from build123d import *

# Parameters (mm, degrees)
SKETCH_1_W          = 40
SKETCH_1_H          = 80
SKETCH_1_R          = 4.25
SKETCH_1_R_2        = 5.1
EXTRUDE_1_DEPTH     = 12
SKETCH_3_R          = 6.5
CUT_EXTRUDE_1_DEPTH = 7
SWEEP_1_PITCH       = 1.75
SWEEP_1_HEIGHT      = 12
SWEEP_1_RADIUS      = 5.1
SWEEP_1_START_ANGLE = 90
SKETCH_6_W          = 42.021889548
SKETCH_6_H          = 2.845778449
SKETCH_6_W_2        = 42.914668854
SKETCH_6_H_2        = 10.152042119
CUT_EXTRUDE_2_DEPTH = 91.331481783


with BuildPart() as part:
    # 草图1 → 凸台-拉伸1 (new body)
    with BuildSketch(Plane(origin=(0, 0, 0), x_dir=(1, 0, 0), z_dir=(0, 1, 0))):
        with Locations((20, 40)):
            Rectangle(SKETCH_1_W, SKETCH_1_H)
        with Locations(Location((20, 60, 0), (0, 0, 270))):
            Circle(SKETCH_1_R, mode=Mode.SUBTRACT)
        with Locations(Location((20, 20, 0), (0, 0, 270))):
            Circle(SKETCH_1_R, mode=Mode.SUBTRACT)
        with Locations(Location((20, 40, 0), (0, 0, 270))):
            Circle(SKETCH_1_R_2, mode=Mode.SUBTRACT)
    extrude(amount=EXTRUDE_1_DEPTH)

    # 草图3 → 切除-拉伸1 (cut)
    with BuildSketch(Plane(origin=(0, 12, 0), x_dir=(1, 0, 0), z_dir=(0, 1, 0))):
        with Locations(Location((20, 20, 0), (0, 0, 270))):
            Circle(SKETCH_3_R)
        with Locations(Location((20, 60, 0), (0, 0, 270))):
            Circle(SKETCH_3_R)
    extrude(amount=-CUT_EXTRUDE_1_DEPTH, mode=Mode.SUBTRACT)

    # 扫描1: sweep along a helix
    with BuildLine() as sweep_1_path:
        add(Helix(SWEEP_1_PITCH, SWEEP_1_HEIGHT, SWEEP_1_RADIUS, center=(20, 12, -40), direction=(0, -1, 0), mode=Mode.PRIVATE).rotate(Axis((20, 12, -40), (0, -1, 0)), SWEEP_1_START_ANGLE))
    # 草图5 → 扫描1 (sweep)
    with BuildSketch(Plane(origin=(25.1, 12, -40), x_dir=(1, 0, 0), z_dir=(5.189082450239955e-15, -0.054530732695540304, 0.9985120926617203))):
        Polygon((-0.740428606, 0), (0.370214303, -0.641229983), (0.370214303, 0.641229983), align=None)
    sweep(path=sweep_1_path.line, is_frenet=True)

    # 草图6 → 切除-拉伸2 (cut, through all)
    with BuildSketch(Plane(origin=(0, 0, -80), x_dir=(-1, 0, 0), z_dir=(0, 0, -1))):
        with Locations((-18.989055226, 13.422889225)):
            Rectangle(SKETCH_6_W, SKETCH_6_H)
        with Locations((-18.542665573, -5.07602106)):
            Rectangle(SKETCH_6_W_2, SKETCH_6_H_2)
    extrude(amount=-CUT_EXTRUDE_2_DEPTH, mode=Mode.SUBTRACT)


solid = part.part
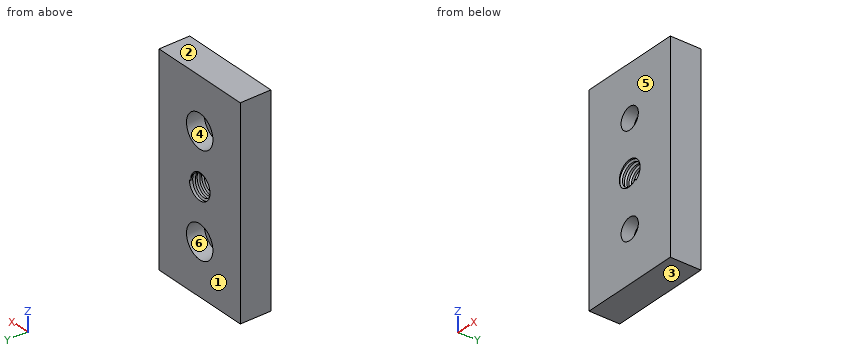
Verification items for the finished model (mm, model axes). Face numbers are marked on the shaded views. A direction names the side the tool comes from. Coordinates: 2 decimals unless noted, no trailing zeros. Write each loop counter-clockwise with the first axis right and the second up, starting at its lowest first coordinate (ties: lowest second). Pieces come first, ordered by that corner, then holes. Notation, with made-up numbers: (-27.5, 79) - (10.5, 79) arc R27 ccw to (10.5, 98) - close; hole circle Ø10 at (-7.5, 27). An arc over 180 degrees is marked (long way). Answer as a JSON object with one key per item and string values.
(1) Mould release check, pull along Z, two halves, no side actions. Record for the marked faces 1, 2, 3 and 4: pulls with the +Z half, pulls with the -Z half, needs draft (parallel to the pull), parting line crosses it, or undercut.
Report:
{"face 1": "needs draft", "face 2": "pulls with the +Z half", "face 3": "pulls with the -Z half", "face 4": "undercut"}
(2) Cross-section at A-A on z = -20. Record the cut outline in (x, y).
Report:
{"outline": "(0, 0) - (15.75, 0) - (15.75, 5) - (13.5, 5) - (13.5, 12) - (0, 12) - close; (24.25, 0) - (40, 0) - (40, 12) - (26.5, 12) - (26.5, 5) - (24.25, 5) - close"}
(3) Thickness scan on line 1 along Z through (x, y) = (20, 1.45); line 2 along Z through (x, y) = (23, 9); line 3 along Z through (x, y) = (14.5, 5.25). Record the ranges inside material, lowest first.
Report:
{"line 1": "-80 to -64.25, -55.75 to -45.1, -34.97 to -24.25, -15.75 to 0", "line 2": "-80 to -65.77, -54.23 to -43.74, -35.88 to -25.77, -14.23 to 0", "line 3": "-80 to -63.46, -56.54 to -23.46, -16.54 to 0"}
(4) Cross-section at B-B on x = 17.5. Give the number of separate pieces and of enclosed holes in the cut face, plus the area to 3 significant figures.
Report:
{"separate pieces": "4", "enclosed holes": "0", "area": "622 mm^2"}
(5) Tool access check on the marked faces 5 and 6. Record the directions out of +Z, -Z, +X, -X, +Y, -Y that give a thin tool (end or side, any length) a straight path to the whole face; none if there is none.
Report:
{"face 5": "+Z, -Z, +X, -X, -Y", "face 6": "+Y"}
(6) Gauge pin test, flat end, axial feed: pin 1 Ø1.5 at (x, z) = (17, -64) entering from +Y. Record the tip position at first contact, or that the pin passes through.
Report:
{"pin 1": "y = 5"}
